Part model, mm, in its own coordinate system. Coordinates: 2 decimals unless noted, no trailing zeros. Loops run counter-clockwise (first coordinate to the right, second up) from the corner with the lowest first, then second, coordinate; pieces in that order, holes last. Notation, with made-up numbers: (-37.75, -40) -> (12.25, -40) arc R4 ccw to (12.25, -36) -> close; hole circle Ø11 at (19, 84.25). An arc over 180 degrees is marked (long way). One line per question, with ' | ' between items. Start each with the question number.
1) Two-plate mould, pull along X, no slides. Class faces 1 (the face through (-20.51, 0.68, -18.38)), 2 (the face through (9, 2, 9)), 3 (the face through (-7, 3, -7)): released by +X, released by -X, zero draft, split by the parting line, or undercut.
2) Cut at A-A (z = 0). List the corners of the cut face in (x, y).
3) Probe L1, parallel to Z at x = -20, y = 0.45; L2, parallel to X at y = 0.65, z = 0. List the from-to ranges inside material, lowest first. Write a range as from..to.
4) Cut at B-B (y = 2.45). List the corners of the cut face in (x, z).
5) Drop flat-ended pins along their axis: pin 1 (1 mm diameter, centred on x = 23.5, y = 2, fed in from +Z); pin 2 (2.5 mm diameter, centred on x = 0, z = -20, fed in from -Y). Give the stop position or say it passes through.
6) Cut at C-C (x = 0). List the corners of the cut face in (y, z), plus the area to 3 significant figures.
7) Cut at D-D (z = -20). List the corners of the cut face in (x, y), plus the area to 3 significant figures.
from build123d import *

# Parameters (mm, degrees)
SKETCH2_W                                    = 60
SKETCH2_H                                    = 60
BOSS_EXTRUDE1_DEPTH                          = 3
CUT_EXTRUDE1_DEPTH                           = 10
CSK_FOR_M3_HEX_SOCKET_COUNTERSUNK_CA_2_COUNT = 2
CSK_FOR_M3_HEX_SOCKET_COUNTERSUNK_CA_2_PITCH = 20
CSK_FOR_M3_HEX_SOCKET_COUNTERSUNK_CA_3_COUNT = 2
CSK_FOR_M3_HEX_SOCKET_COUNTERSUNK_CA_3_PITCH = 40
CSK_FOR_M3_HEX_SOCKET_COUNTERSUNK_CA_4_COUNT = 2
CSK_FOR_M3_HEX_SOCKET_COUNTERSUNK_CA_4_PITCH = 20
CSK_FOR_M3_HEX_SOCKET_COUNTERSUNK_CA_5_COUNT = 2
CSK_FOR_M3_HEX_SOCKET_COUNTERSUNK_CA_5_PITCH = 40
FILLET1_R                                    = 1


with BuildPart() as part:
    # Sketch2 → Boss-Extrude1 (new body)
    with BuildSketch(Plane(origin=(0, 0, 0), x_dir=(1, 0, 0), z_dir=(0, 1, 0))):
        Rectangle(SKETCH2_W, SKETCH2_H)
    extrude(amount=BOSS_EXTRUDE1_DEPTH)

    # Sketch3 → Cut-Extrude1 (cut)
    with BuildSketch(Plane(origin=(0, 3, 0), x_dir=(1, 0, 0), z_dir=(0, 1, 0))):
        Polygon((30, 12), (-12, -30), (30, -30), align=None)
    extrude(amount=-CUT_EXTRUDE1_DEPTH, mode=Mode.SUBTRACT)

    # Sketch6 → CSK for M3 Hex Socket Countersunk Cap Screw1 (revolve, cut)
    with BuildSketch(Plane(origin=(-20, 3, -20), x_dir=(0, 0, 1), z_dir=(1, 0, 0))):
        Polygon((0, 0), (0, 3), (1.7, 3), (1.7, 1.66), (3.36, 0), align=None)
    csk_for_m3_hex_socket_countersunk_cap_sc = revolve(axis=Axis((-20, 9.35, -20), (0, -1, 0)), mode=Mode.SUBTRACT)

    # CSK for M3 Hex Socket Countersunk Ca 2: CSK for M3 Hex Socket Countersunk Cap Screw1 ×2
    with Locations(*[(i * CSK_FOR_M3_HEX_SOCKET_COUNTERSUNK_CA_2_PITCH, 0, 0) for i in range(1, CSK_FOR_M3_HEX_SOCKET_COUNTERSUNK_CA_2_COUNT)]):
        add(csk_for_m3_hex_socket_countersunk_cap_sc, mode=Mode.SUBTRACT)

    # CSK for M3 Hex Socket Countersunk Ca 3: CSK for M3 Hex Socket Countersunk Cap Screw1 ×2
    with Locations(*[(i * CSK_FOR_M3_HEX_SOCKET_COUNTERSUNK_CA_3_PITCH, 0, 0) for i in range(1, CSK_FOR_M3_HEX_SOCKET_COUNTERSUNK_CA_3_COUNT)]):
        add(csk_for_m3_hex_socket_countersunk_cap_sc, mode=Mode.SUBTRACT)

    # CSK for M3 Hex Socket Countersunk Ca 4: CSK for M3 Hex Socket Countersunk Cap Screw1 ×2
    with Locations(*[(0, 0, i * CSK_FOR_M3_HEX_SOCKET_COUNTERSUNK_CA_4_PITCH) for i in range(1, CSK_FOR_M3_HEX_SOCKET_COUNTERSUNK_CA_4_COUNT)]):
        add(csk_for_m3_hex_socket_countersunk_cap_sc, mode=Mode.SUBTRACT)

    # CSK for M3 Hex Socket Countersunk Ca 5: CSK for M3 Hex Socket Countersunk Cap Screw1 ×2
    with Locations(*[(0, 0, i * CSK_FOR_M3_HEX_SOCKET_COUNTERSUNK_CA_5_PITCH) for i in range(1, CSK_FOR_M3_HEX_SOCKET_COUNTERSUNK_CA_5_COUNT)]):
        add(csk_for_m3_hex_socket_countersunk_cap_sc, mode=Mode.SUBTRACT)

    # Fillet1
    fillet1_edges = [part.edges().sort_by_distance(p)[0] for p in [
        (30, 1.5, -12),
        (-12, 1.5, 30),
        (-30, 1.5, 30),
        (-30, 1.5, -30),
        (30, 1.5, -30),
    ]]
    fillet(fillet1_edges, radius=FILLET1_R)


solid = part.part
Reported:
1) face 1: undercut | face 2: released by +X | face 3: zero draft
2) outline: (-30, 0) -> (-21.7, 0) -> (-21.7, 1.34) -> (-23.36, 3) -> (-30, 3) -> close; (-18.3, 0) -> (18, 0) -> (18, 3) -> (-16.64, 3) -> (-18.3, 1.34) -> close
3) L1: z = -30..-21.7, -18.3..-1.7, 1.7..18.3, 21.7..30 | L2: x = -30..-21.7, -18.3..18
4) outline: (-30, -29) arc R1 ccw to (-29, -30) -> (29, -30) arc R1 ccw to (30, -29) -> (30, -12.41) arc R1 ccw to (29.71, -11.71) -> (-11.71, 29.71) arc R1 ccw to (-12.41, 30) -> (-29, 30) arc R1 ccw to (-30, 29) -> close; hole circle Ø5.62 at (-20, -20); hole circle Ø5.62 at (-20, 0); hole circle Ø5.62 at (-20, 20); hole circle Ø5.62 at (0, -20); hole circle Ø5.62 at (20, -20)
5) pin 1: stops at z = -5 | pin 2: passes through
6) outline: (0, -30) -> (3, -30) -> (3, -23.36) -> (1.34, -21.7) -> (0, -21.7) -> close; (0, -18.3) -> (1.34, -18.3) -> (3, -16.64) -> (3, 18) -> (0, 18) -> close | area: 131 mm²
7) outline: (-30, 0) -> (-21.7, 0) -> (-21.7, 1.34) -> (-23.36, 3) -> (-30, 3) -> close; (-18.3, 0) -> (-1.7, 0) -> (-1.7, 1.34) -> (-3.36, 3) -> (-16.64, 3) -> (-18.3, 1.34) -> close; (1.7, 0) -> (18.3, 0) -> (18.3, 1.34) -> (16.64, 3) -> (3.36, 3) -> (1.7, 1.34) -> close; (21.7, 0) -> (30, 0) -> (30, 3) -> (23.36, 3) -> (21.7, 1.34) -> close | area: 141 mm²
